Geometry check sheet. Reference: the model listing, model coordinates, mm. Face numbers are marked on the shaded views. Coordinates: 2 decimals unless noted, no trailing zeros. Order: outer loops, then holes, each group sorted by start corner. A loop starts at its lowest first (then second) coordinate and runs counter-clockwise, first axis right, second up. Notation, with made-up numbers: (43, 37) -> (80, 37) arc R14 ccw to (80, 59) -> close; hole circle Ø4 at (-18, -11). An arc over 180 degrees is marked (long way). Answer as CSV lines item,"result". Start each with the question number.
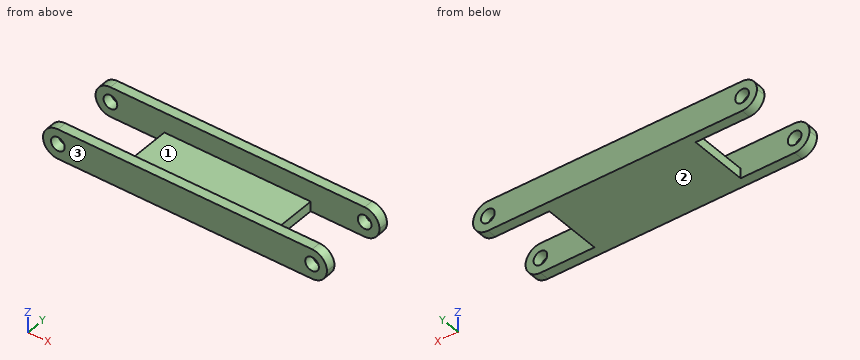
from build123d import *

# Parameters (mm, degrees)
F0_W     = 15
F0_H     = 2.5
F1_DEPTH = 18.7
F2_DEPTH = 36.3
F3_R     = 1.75
F4_DEPTH = 20.001


with BuildPart() as f1:
    # F0 (on Right) → F1 (new body, symmetric)
    with BuildSketch(Plane.YZ):
        with Locations((0, 1.25)):
            Rectangle(F0_W, F0_H)
    extrude(amount=F1_DEPTH, both=True)

    # F0 (on Right) → F2 (join, symmetric)
    with BuildSketch(Plane.YZ):
        Polygon((-10, 0), (-7.5, 0), (-7.5, 2.5), (-7.5, 7.6), (-10, 7.6), align=None)
        Polygon((7.5, 2.5), (7.5, 0), (10, 0), (10, 7.6), (7.5, 7.6), align=None)
    extrude(amount=F2_DEPTH, both=True)

    # F3 (on face) → F4 (cut, through all)
    with BuildSketch(Plane.XZ.offset(10)):
        with Locations((-32.5, 3.8)):
            Circle(F3_R)
        with Locations((32.5, 3.8)):
            Circle(F3_R)
        Polygon((-36.3, 0), (-36.3, 3.8), (-36.3, 7.6), (-40.478576, 7.6), (-40.478576, 0), align=None)
        with BuildLine():
            Line((-36.3, 0), (-32.5, 0))
            ThreePointArc((-32.5, 0), (-35.187006, 1.112994), (-36.3, 3.8))
            Line((-36.3, 3.8), (-36.3, 0))
        make_face()
        with BuildLine():
            ThreePointArc((-36.3, 3.8), (-35.187006, 6.487006), (-32.5, 7.6))
            Line((-32.5, 7.6), (-36.3, 7.6))
            Line((-36.3, 7.6), (-36.3, 3.8))
        make_face()
        with BuildLine():
            Line((36.3, 7.6), (32.5, 7.6))
            ThreePointArc((32.5, 7.6), (35.187006, 6.487006), (36.3, 3.8))
            Line((36.3, 3.8), (36.3, 7.6))
        make_face()
        with BuildLine():
            ThreePointArc((36.3, 3.8), (35.187006, 1.112994), (32.5, 0))
            Line((32.5, 0), (36.3, 0))
            Line((36.3, 0), (36.3, 3.8))
        make_face()
        Polygon((40.478576, 7.6), (36.3, 7.6), (36.3, 3.8), (36.3, 0), (40.478576, 0), align=None)
    extrude(amount=-F4_DEPTH, mode=Mode.SUBTRACT)


solid = f1.part
Q1. Sectioned sample at B-B, the plane y = -5.25. Record the cut outline in (x, z).
Q2. Thickness scan on L1, parallel to Z at x = -32.5, y = 8.25; L2, parallel to X at y = -8.75, z = 3.75; L3, parallel to Y at x = -6, z = 4.5. Record the ranges inside material, lowest first.
Q3. Sectioned sample at A-A, the plane x = 3. Record the cut outline in (y, z).
Q4. Release check for a two-part mould opening along Y. For the marked faces 1, 2 and 3 record: released by +Y, released by -Y, zero draft, split by the parting line, or undercut.
Q5. Go/stop test with flat-tipped pins: pin 1 Ø0.8 at (y, z) = (-2, 1.5) entering from +X; pin 2 Ø2 at (x, z) = (32.5, 3.8) entering from +Y; pin 3 Ø7.5 at (x, y) = (-2, -3) entering from +Z; pin 4 Ø2 at (y, z) = (2.5, 1) entering from -X. Record where each tip stops, or that it passes through.
Geometry results:
1,outline,"(-18.7, 0) -> (18.7, 0) -> (18.7, 2.5) -> (-18.7, 2.5) -> close"
2,L1,"z = 0 to 2.05, 5.55 to 7.6"
2,L2,"x = -36.3 to -34.25, -30.75 to 30.75, 34.25 to 36.3"
2,L3,"y = -10 to -7.5, 7.5 to 10"
3,outline,"(-10, 0) -> (10, 0) -> (10, 7.6) -> (7.5, 7.6) -> (7.5, 2.5) -> (-7.5, 2.5) -> (-7.5, 7.6) -> (-10, 7.6) -> close"
4,face 1,"undercut"
4,face 2,"zero draft"
4,face 3,"released by -Y"
5,pin 1,"stops at x = 18.7"
5,pin 2,"passes through"
5,pin 3,"stops at z = 2.5"
5,pin 4,"stops at x = -18.7"
